Check sheet for the modelled part. Datum: model origin and axes. Units: mm. Face numbers are marked on the shaded views. A direction names the side the tool comes from. Give positions to 0.01 mm unless a question says otherwise; leave off trailing zeros. Order: outer loops, then holes, each group sorted by start corner. A loop starts at its lowest first (then second) coordinate and runs counter-clockwise, first axis right, second up.
```python
from build123d import *

# Parameters (mm, degrees)
BOSS_EXTRUDE1_DEPTH = 40
SKETCH3_R           = 2.5
BOSS_EXTRUDE2_DEPTH = 5
BOSS_EXTRUDE3_DEPTH = 30
SKETCH5_R           = 17.5
SKETCH5_R_2         = 15.5
SKETCH5_R_3         = 9.5
SKETCH5_R_4         = 7.5
CUT_EXTRUDE1_DEPTH  = 1


with BuildPart() as part:
    # Sketch1 → Boss-Extrude1 (new body)
    with BuildSketch(Plane.XY):
        Polygon((-27.5, -17.5), (-27.5, 17.5), (-17.5, 17.5), (-17.5, 27.5), (17.5, 27.5), (17.5, 17.5), (27.5, 17.5), (27.5, -17.5), (17.5, -17.5), (17.5, -27.5), (-17.5, -27.5), (-17.5, -17.5), align=None)
    extrude(amount=BOSS_EXTRUDE1_DEPTH)

    # Sketch3 → Boss-Extrude2 (add)
    # profile 1 of 5: a face of its own
    with BuildSketch(Plane.XY.offset(40)):
        Polygon((17.5, 27.5), (-17.5, 27.5), (-17.5, 17.5), (-27.5, 17.5), (-27.5, -17.5), (-17.5, -17.5), (-17.5, -27.5), (17.5, -27.5), (17.5, -17.5), (27.5, -17.5), (27.5, 17.5), (17.5, 17.5), align=None)
    # profile 2 of 5: a face of its own
    with BuildSketch(Plane.XY.offset(40)):
        with BuildLine():
            Line((24.5, 27.5), (17.5, 27.5))
            Line((17.5, 27.5), (17.5, 17.5))
            Line((17.5, 17.5), (27.5, 17.5))
            Line((27.5, 17.5), (27.5, 24.5))
            ThreePointArc((27.5, 24.5), (26.621320344, 26.621320344), (24.5, 27.5))
        make_face()
        with Locations((23, 23)):
            Circle(SKETCH3_R, mode=Mode.SUBTRACT)
    # profile 3 of 5: a face of its own
    with BuildSketch(Plane.XY.offset(40)):
        with BuildLine():
            Line((27.5, -24.5), (27.5, -17.5))
            Line((27.5, -17.5), (17.5, -17.5))
            Line((17.5, -17.5), (17.5, -27.5))
            Line((17.5, -27.5), (24.5, -27.5))
            ThreePointArc((24.5, -27.5), (26.621320344, -26.621320344), (27.5, -24.5))
        make_face()
        with Locations((23, -23)):
            Circle(SKETCH3_R, mode=Mode.SUBTRACT)
    # profile 4 of 5: a face of its own
    with BuildSketch(Plane.XY.offset(40)):
        with BuildLine():
            Line((-17.5, -17.5), (-27.5, -17.5))
            Line((-27.5, -17.5), (-27.5, -24.5))
            ThreePointArc((-27.5, -24.5), (-26.621320344, -26.621320344), (-24.5, -27.5))
            Line((-24.5, -27.5), (-17.5, -27.5))
            Line((-17.5, -27.5), (-17.5, -17.5))
        make_face()
        with Locations((-23, -23)):
            Circle(SKETCH3_R, mode=Mode.SUBTRACT)
    # profile 5 of 5: a face of its own
    with BuildSketch(Plane.XY.offset(40)):
        with BuildLine():
            Line((-17.5, 17.5), (-17.5, 27.5))
            Line((-17.5, 27.5), (-24.5, 27.5))
            ThreePointArc((-24.5, 27.5), (-26.621320344, 26.621320344), (-27.5, 24.5))
            Line((-27.5, 24.5), (-27.5, 17.5))
            Line((-27.5, 17.5), (-17.5, 17.5))
        make_face()
        with Locations((-23, 23)):
            Circle(SKETCH3_R, mode=Mode.SUBTRACT)
    extrude(amount=-BOSS_EXTRUDE2_DEPTH)

    # Sketch4 → Boss-Extrude3 (add)
    with BuildSketch(Plane.XY.offset(40)):
        with BuildLine():
            ThreePointArc((5, 0), (3.535533906, 3.535533906), (0, 5))
            Line((0, 5), (0, -5))
            ThreePointArc((0, -5), (3.535533906, -3.535533906), (5, 0))
        make_face()
        with BuildLine():
            Line((0, -5), (0, 5))
            ThreePointArc((0, 5), (-5, 0), (0, -5))
        make_face()
    extrude(amount=BOSS_EXTRUDE3_DEPTH)

    # Sketch5 → Cut-Extrude1 (cut)
    # profile 1 of 2: a face of its own
    with BuildSketch(Plane.XY.offset(40)):
        Circle(SKETCH5_R)
        Circle(SKETCH5_R_2, mode=Mode.SUBTRACT)
    # profile 2 of 2: a face of its own
    with BuildSketch(Plane.XY.offset(40)):
        Circle(SKETCH5_R_3)
        Circle(SKETCH5_R_4, mode=Mode.SUBTRACT)
    extrude(amount=-CUT_EXTRUDE1_DEPTH, mode=Mode.SUBTRACT)


solid = part.part
```
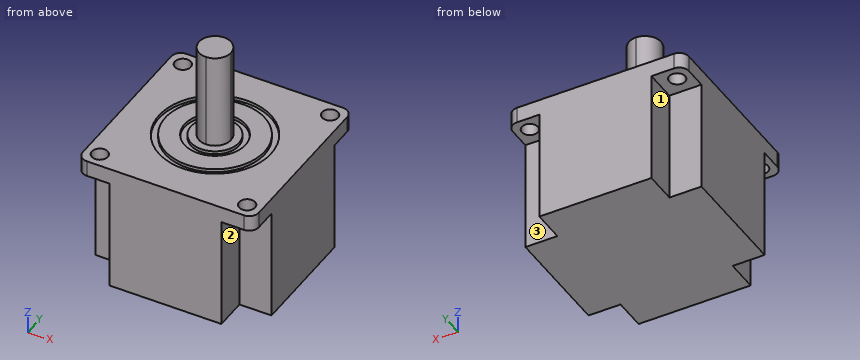
(1) Cross-section at B-B on y = -23. Enter the section's corners in (x, z), then the cut area to 3 significant figures.
Response values:
outline: (-27.5, 35) - (-25.5, 35) - (-25.5, 40) - (-27.5, 40) - close; (-20.5, 35) - (-17.5, 35) - (-17.5, 0) - (17.5, 0) - (17.5, 35) - (20.5, 35) - (20.5, 40) - (-20.5, 40) - close; (25.5, 35) - (27.5, 35) - (27.5, 40) - (25.5, 40) - close
area: 1,450 mm2
(2) Gauge pin test, flat ends, axial feed: pin 1 Ø6.5 at (x, y) = (-23, -23) entering from -Z; pin 2 Ø3 at (y, z) = (24.5, 21) entering from -X; pin 3 Ø2 at (x, y) = (-16.5, 15) entering from +Z. Record the tip position at first contact, or that the pin passes through.
Response values:
pin 1: stops at z = 35
pin 2: stops at x = -17.5
pin 3: stops at z = 40
(3) Set-up check for the marked faces 1, 2 and 3: record each of +Z, -Z, +X, -X, +Y, -Y from which the full face is reachable in a straight line by a thin tool's end or side.
Response values:
face 1: -Z, -X, +Y
face 2: -Z, +X, -Y
face 3: -Z, +X, +Y
(4) Material ranges on L1, parallel to Y at x = 23, z = 36.9; L2, parallel to Y at x = 0, z = 39.3; L3, parallel to Y at x = -6, z = 39.5, recorded low to high.
Response values:
L1: y = -27.5 to -25.5, -20.5 to 20.5, 25.5 to 27.5
L2: y = -27.5 to -17.5, -15.5 to -9.5, -7.5 to 7.5, 9.5 to 15.5, 17.5 to 27.5
L3: y = -27.5 to -16.44, -14.29 to -7.37, -4.5 to 4.5, 7.37 to 14.29, 16.44 to 27.5
(5) Cross-section at D-D on x = 8.5. Enter the section's corners in (y, z), then the cut area to 3 significant figures.
Response values:
outline: (-27.5, 0) - (27.5, 0) - (27.5, 40) - (15.3, 40) - (15.3, 39) - (12.96, 39) - (12.96, 40) - (4.24, 40) - (4.24, 39) - (-4.24, 39) - (-4.24, 40) - (-12.96, 40) - (-12.96, 39) - (-15.3, 39) - (-15.3, 40) - (-27.5, 40) - close
area: 2,190 mm2
(6) Cross-section at A-A on x = -21.5. Enter the section's corners in (y, z), then the cut area to 3 significant figures.
Response values:
outline: (-27.5, 35) - (-25, 35) - (-25, 40) - (-27.5, 40) - close; (-21, 35) - (-17.5, 35) - (-17.5, 0) - (17.5, 0) - (17.5, 35) - (21, 35) - (21, 40) - (-21, 40) - close; (25, 35) - (27.5, 35) - (27.5, 40) - (25, 40) - close
area: 1,460 mm2
(7) Cross-section at C-C on y = -12.5. Enter the section's corners in (x, z).
Response values:
outline: (-27.5, 0) - (27.5, 0) - (27.5, 40) - (12.25, 40) - (12.25, 39) - (9.17, 39) - (9.17, 40) - (-9.17, 40) - (-9.17, 39) - (-12.25, 39) - (-12.25, 40) - (-27.5, 40) - close
